from build123d import *

# Parameters (mm, degrees)
SKETCH1_R           = 15
BOSS_EXTRUDE1_DEPTH = 210
CHAMFER1_SIZE       = 2
CHAMFER2_SIZE       = 3
CHAMFER2_SIZE2      = 11.196152423


with BuildPart() as part:
    # Sketch1 → Boss-Extrude1 (new body)
    with BuildSketch(Plane(origin=(0, 0, 0), x_dir=(1, 0, 0), z_dir=(0, 1, 0))):
        with Locations(Location((0, 0, 0), (0, 0, 270))):
            Circle(SKETCH1_R)
    extrude(amount=-BOSS_EXTRUDE1_DEPTH)

    # Chamfer1
    chamfer1_edges = [part.edges().sort_by_distance(p)[0] for p in [
        (0, -210, -15),
    ]]
    chamfer(chamfer1_edges, length=CHAMFER1_SIZE)

    # Chamfer2
    chamfer2_edges = [part.edges().sort_by_distance(p)[0] for p in [
        (0, 0, -15),
    ]]
    chamfer2_side = [part.faces().sort_by_distance(p)[0] for p in [
        (0, 0, 0),
    ]]
    chamfer(chamfer2_edges, length=CHAMFER2_SIZE, length2=CHAMFER2_SIZE2, reference=chamfer2_side[0])


solid = part.part
Geometry check sheet. Reference: the model listing, model coordinates, mm. Give positions to 0.01 mm unless a question says otherwise; leave off trailing zeros. Order: outer loops, then holes, each group sorted by start corner. A loop starts at its lowest first (then second) coordinate and runs counter-clockwise, first axis right, second up.
1) Gauge pin test, flat ends, axial feed: pin 1 (5 mm diameter, centred on y = -22.5, z = -11.5, fed in from -X); pin 2 (5 mm diameter, centred on y = -48, z = -7.5, fed in from +X); pin 3 (10 mm diameter, centred on y = -84.5, z = 2.5, fed in from +X); pin 4 (1 mm diameter, centred on x = -7, y = -31, fed in from -Z). Record the tip position at first contact, or that the pin passes through.
Results are:
pin 1: stops at x = -12
pin 2: stops at x = 14.14
pin 3: stops at x = 15
pin 4: stops at z = -13.52
2) Cross-section at A-A (y = -21.5). Record the boundary of the cut face in (x, z), then the cut area to 3 significant figures.
Results are:
outline: circle Ø30 at (0, 0)
area: 707 mm2
3) Material ranges on probe 1 along X at (y, z) = (-100, -0.75); probe 2 along Z at (x, y) = (1, -112); probe 3 along Z at (x, y) = (-7.5, -78), recorded low to high.
Results are:
probe 1: x = -14.98 to 14.98
probe 2: z = -14.97 to 14.97
probe 3: z = -12.99 to 12.99
